Input: part model. Units: mm. Frame: model coordinates. A direction names the side the tool comes from. Coordinates: 2 decimals unless noted, no trailing zeros. Write each loop counter-clockwise with the first axis right and the second up, starting at its lowest first coordinate (ties: lowest second). Pieces come first, ordered by that corner, then holes.
from build123d import *

# Parameters (mm, degrees)
BOX003_W                  = 5
BOX003_H                  = 2
BOX003_DEPTH              = 5
BOX005_W                  = 5
BOX005_H                  = 2
BOX005_DEPTH              = 5
BOX002_W                  = 17
BOX002_H                  = 33
BOX002_DEPTH              = 5
BOX001_W                  = 20
BOX001_H                  = 36
BOX001_DEPTH              = 5
BOX_W                     = 21.8
BOX_H                     = 41.8
BOX_DEPTH                 = 1.5
FUSION004_PLACEMENT_ANGLE = 180


with BuildPart() as cube001:
    # Box003 → Box003 (new body)
    with BuildSketch(Plane(origin=(-10, 17.4, 0), x_dir=(1, 0, 0), z_dir=(0, 0, 1))):
        with Locations((2.5, 1)):
            Rectangle(BOX003_W, BOX003_H)
    extrude(amount=BOX003_DEPTH)


with BuildPart() as fusion003:
    # Box005 → Box005 (new body)
    with BuildSketch(Plane(origin=(-10, -19.4, 0), x_dir=(1, 0, 0), z_dir=(0, 0, 1))):
        with Locations((2.5, 1)):
            Rectangle(BOX005_W, BOX005_H)
    extrude(amount=BOX005_DEPTH)

    # Fusion003: union Cube001
    add(cube001.part)


with BuildPart() as fusion003_1:
    # Fusion003 placement: moved
    add(fusion003.part.moved(Location((15, 0, 0))))


with BuildPart() as cut:
    # Box002 → Box002 (new body)
    with BuildSketch(Plane(origin=(-8.5, -16.5, 0), x_dir=(1, 0, 0), z_dir=(0, 0, 1))):
        with Locations((8.5, 16.5)):
            Rectangle(BOX002_W, BOX002_H)
    extrude(amount=BOX002_DEPTH)


with BuildPart() as cube:
    # Box001 → Box001 (new body)
    with BuildSketch(Plane(origin=(-10, -18, 0), x_dir=(1, 0, 0), z_dir=(0, 0, 1))):
        with Locations((10, 18)):
            Rectangle(BOX001_W, BOX001_H)
    extrude(amount=BOX001_DEPTH)


with BuildPart() as basesensoruppermount:
    # Box → Box (new body)
    with BuildSketch(Plane(origin=(-10.9, -20.9, 0), x_dir=(1, 0, 0), z_dir=(0, 0, 1))):
        with Locations((10.9, 20.9)):
            Rectangle(BOX_W, BOX_H)
    extrude(amount=BOX_DEPTH)

    # Fusion: union Cube
    add(cube.part)

    # Cut: cut cut
    add(cut.part, mode=Mode.SUBTRACT)

    # Fusion004: union Fusion003
    add(fusion003_1.part)


with BuildPart() as basesensoruppermount_1:
    # Fusion004 placement: moved
    add(basesensoruppermount.part.moved(Location((0, 0, 1.5))).rotate(Axis((0, 0, 1.5), (0, 1, 0)), FUSION004_PLACEMENT_ANGLE))


solid = basesensoruppermount_1.part
Item 1: Section query B-B, the plane z = -2.75. Return loops of the section in (x, y), then the cut area to 3 significant figures.
Item 2: Pull-direction query (X, two-part tool) for faces 1 (the face through (-10.9, 0, 1)), 2 (the face through (0, 16.5, -1)), 3 (the face through (3, -18, -2)); classes: released by +X, released by -X, zero draft, split by the parting line, or undercut.
Item 3: Access query for faces 4 (the face through (3, 18, -2)), 5 (the face through (-7, -19.4, -2)), 6 (the face through (-10, 0, -2)), 7 (the face through (0, -16.5, -1)). Directions: +Z, -Z, +X, -X, +Y, -Y. A direction counts if a zero-diameter tool reaches every point of the face in a straight line with its end or side. Return the directions, or none.
Item 4: Material intervals for line 1 (X direction, y = -14.5, z = -2.2); line 2 (Y direction, x = 6.75, z = 0.2); line 3 (Y direction, x = 8.25, z = -0.6), sorted ascending.
Item 5: Section query C-C, the plane y = -13.5. Return loops of the section in (x, z), then the cut area to 3 significant figures.
Item 6: Pin query (flat end, axial travel): pin 1 Ø2.5 at (y, z) = (6.5, -2) entering from +X; pin 2 Ø4 at (x, y) = (-6, 2) entering from -Z. Return the tip coordinate at first contact, or that it passes through.
Item 7: Section query A-A, the plane x = -7. Return loops of the section in (y, z).
Item 8: Section query D-D, the plane x = 9. Return loops of the section in (y, z), then the cut area to 3 significant figures.
The answers:
1. outline: (-10, -19.4) - (-5, -19.4) - (-5, -18) - (10, -18) - (10, 18) - (-5, 18) - (-5, 19.4) - (-10, 19.4) - close; hole (-8.5, -16.5) - (8.5, -16.5) - (8.5, 16.5) - (-8.5, 16.5) - close
1. area: 173 mm2
2. face 1: released by -X
2. face 2: undercut
2. face 3: zero draft
3. face 4: -Z, +X, +Y
3. face 5: -Z, +X, -X, -Y
3. face 6: -Z, -X, +Y, -Y
3. face 7: +Z, -Z
4. line 1: x = -10 to -8.5, 8.5 to 10
4. line 2: y = -20.9 to -16.5, 16.5 to 20.9
4. line 3: y = -18 to -16.5, 16.5 to 18
5. outline: (-10.9, 0) - (-10, 0) - (-10, -3.5) - (-8.5, -3.5) - (-8.5, 1.5) - (-10.9, 1.5) - close; (8.5, -3.5) - (10, -3.5) - (10, 0) - (10.9, 0) - (10.9, 1.5) - (8.5, 1.5) - close
5. area: 17.7 mm2
6. pin 1: stops at x = 10
6. pin 2: passes through
7. outline: (-20.9, 0) - (-19.4, 0) - (-19.4, -3.5) - (-16.5, -3.5) - (-16.5, 1.5) - (-20.9, 1.5) - close; (16.5, -3.5) - (19.4, -3.5) - (19.4, 0) - (20.9, 0) - (20.9, 1.5) - (16.5, 1.5) - close
8. outline: (-20.9, 0) - (-18, 0) - (-18, -3.5) - (18, -3.5) - (18, 0) - (20.9, 0) - (20.9, 1.5) - (-20.9, 1.5) - close
8. area: 189 mm2
